The model under review builds one solid part; all positions refer to its coordinate system, in mm. Give positions to 0.01 mm unless a question says otherwise; leave off trailing zeros. Write each loop counter-clockwise with the first axis right and the second up, starting at its lowest first coordinate (ties: lowest second). Pieces come first, ordered by that corner, then holes. Notation, with made-up numbers: (-36, -19) -> (17, -19) arc R20 ccw to (17, 9) -> close; hole circle Ø6 at (-10.5, -7). An arc over 180 degrees is marked (long way). Use CSV: the item, a comma, the result in double quotes.
```python
from build123d import *

# Parameters (mm, degrees)
ESBO_O1_W             = 51
ESBO_O1_H             = 12.7
FLANGE_BASE1_DEPTH    = 3.18
ESBO_O2_R             = 3.5
ESBO_O2_R_2           = 2.25
CORTE_EXTRUS_O1_DEPTH = 10


# Sheet-metal steps are written as plain solids
with BuildPart() as part:
    # Esboço1 → Flange-base1 (new body)
    with BuildSketch(Plane.XY):
        Rectangle(ESBO_O1_W, ESBO_O1_H)
    extrude(amount=-FLANGE_BASE1_DEPTH)

    # Esboço2 → Corte-extrusão1 (cut)
    with BuildSketch(Plane(origin=(0, 0, -3.18), x_dir=(-1, 0, 0), z_dir=(0, 0, -1))):
        with Locations((17.485, 0)):
            Circle(ESBO_O2_R)
        with Locations((-19.4825, 0)):
            Circle(ESBO_O2_R_2)
    extrude(amount=-CORTE_EXTRUS_O1_DEPTH, mode=Mode.SUBTRACT)


solid = part.part
```
Q1. Consider section C-C (z = -2.3). State how many separate pieces and enclosed holes the cut face has, then the cut area to 3 significant figures.
Derived:
separate pieces,"1"
enclosed holes,"2"
area,"593 mm2"
Q2. Consider section A-A (y = 0). Write out the cut boundary in (x, z) (1 decimal).
Derived:
outline,"(-25.5, -3.2) -> (-21, -3.2) -> (-21, 0) -> (-25.5, 0) -> close; (-14, -3.2) -> (17.2, -3.2) -> (17.2, 0) -> (-14, 0) -> close; (21.7, -3.2) -> (25.5, -3.2) -> (25.5, 0) -> (21.7, 0) -> close"
Q3. To check wall thickness, follow probe 1 along X at (y, z) = (-0.25, -2.4); probe 2 along X at (y, z) = (0.5, -0.35); probe 3 along X at (y, z) = (-2.5, -3.05). State the ranges of each line that lie inside material, in increasing order.
Derived:
probe 1,"x = -25.5 to -20.98, -13.99 to 17.25, 21.72 to 25.5"
probe 2,"x = -25.5 to -20.95, -14.02 to 17.29, 21.68 to 25.5"
probe 3,"x = -25.5 to -19.93, -15.04 to 25.5"
Q4. Consider section B-B (x = 20). Write out the cut boundary in (y, z), then the cut area to 3 significant figures.
Derived:
outline,"(-6.35, -3.18) -> (-2.19, -3.18) -> (-2.19, 0) -> (-6.35, 0) -> close; (2.19, -3.18) -> (6.35, -3.18) -> (6.35, 0) -> (2.19, 0) -> close"
area,"26.5 mm2"
Q5. The part is to be moulded in two halves that separate along Y. For faces 1 (the flat face through (-25.5, 0, -2)), 2 (the cylindrical face through (21.73, 0.1, -1.61)), 3 (the flat face through (0, 6.35, -2)), say which applies: pulls with the +Y half, pulls with the -Y half, needs draft (parallel to the pull), parting line crosses it, or undercut.
Derived:
face 1,"needs draft"
face 2,"undercut"
face 3,"pulls with the +Y half"
